```python
from build123d import *

# Parameters (mm, degrees)
SZKIC1_R                    = 85
SZKIC1_R_2                  = 70
DODANIE_WYCI_GNI_CIE1_DEPTH = 10
WYTNIJ_WYCI_GNI_CIE1_START  = -10
SZKIC2_R                    = 3.4
WYTNIJ_WYCI_GNI_CIE1_DEPTH  = 10
SZYK_KO_OWY1_COUNT          = 4


with BuildPart() as part:
    # Szkic1 → Dodanie-wyciągnięcie1 (new body)
    with BuildSketch(Plane.XY):
        Circle(SZKIC1_R)
        Circle(SZKIC1_R_2, mode=Mode.SUBTRACT)
    extrude(amount=DODANIE_WYCI_GNI_CIE1_DEPTH)

    # Szkic2 → Wytnij-wyciągnięcie1 (cut)
    with BuildSketch(Plane.XY.offset(10).offset(WYTNIJ_WYCI_GNI_CIE1_START)):
        with Locations((0, 77.5)):
            Circle(SZKIC2_R)
        with BuildLine():
            Line((-56.196738148, 53.368311023), (-61.501649853, 58.673222728))
            ThreePointArc((-61.501649853, 58.673222728), (-60.104076401, 60.104076401), (-58.673222728, 61.501649853))
            Line((-58.673222728, 61.501649853), (-53.368311023, 56.196738148))
            ThreePointArc((-53.368311023, 56.196738148), (-54.800775542, 54.800775542), (-56.196738148, 53.368311023))
        make_face()
    wytnij_wyci_gni_cie1 = extrude(amount=WYTNIJ_WYCI_GNI_CIE1_DEPTH, mode=Mode.SUBTRACT)

    # Szyk kołowy1: Wytnij-wyciągnięcie1 ×4 about axis
    szyk_ko_owy1_axis = Axis((0, 0, 0), (0, 0, 1))
    for i in range(1, SZYK_KO_OWY1_COUNT):
        add(wytnij_wyci_gni_cie1.rotate(szyk_ko_owy1_axis, i * 360 / SZYK_KO_OWY1_COUNT), mode=Mode.SUBTRACT)


solid = part.part
```
Geometry: final body of the model. Coordinates: model frame, mm. A direction names the side the tool comes from. Coordinates: 2 decimals unless noted, no trailing zeros. Order: outer loops, then holes, each group sorted by start corner. A loop starts at its lowest first (then second) coordinate and runs counter-clockwise, first axis right, second up.
Item 1: Contact query for flat-ended pins moving along their axis: P1, Ø6, axis at x = -60, z = 8.5, coming from the +Y side; P2, Ø2, axis at y = 39.5, z = 1, coming from the -X side; P3, Ø1, axis at x = 48, z = 3.5, coming from the -Y side; P4, Ø8, axis at x = -63, y = 6.5, coming from the -Z side. Output: stop coordinate, or through.
Answer:
P1: stops at y = 63.06
P2: stops at x = -75.78
P3: stops at y = -70.49
P4: passes through
Item 2: Section query D-D (x = -37). Output: boundary loops of the cut face in (y, z), then the cut area to 3 significant figures.
Answer:
outline: (-76.52, 0) - (-59.42, 0) - (-59.42, 10) - (-76.52, 10) - close; (59.42, 0) - (76.52, 0) - (76.52, 10) - (59.42, 10) - close
area: 342 mm2
Item 3: Access query for faces 4 (the face through (-56.06, 58.89, 4.93)), 5 (the face through (84.995, -0.907, 4.93)). Directions: +Z, -Z, +X, -X, +Y, -Y. A direction counts if a zero-diameter tool reaches every point of the face in a straight line with its end or side. Return the directions, or none.
Answer:
face 4: +Z, -Z
face 5: +Z, -Z, +X
Item 4: Material intervals for line 1 along Y through (x, z) = (0, 5); line 2 along Y through (x, z) = (3, 7.5); line 3 along X through (y, z) = (-61, 7.5), sorted ascending.
Answer:
line 1: y = -85 to -80.9, -74.1 to -70, 70 to 74.1, 80.9 to 85
line 2: y = -84.95 to -79.1, -75.9 to -69.94, 69.94 to 75.9, 79.1 to 84.95
line 3: x = -58.17 to -34.34, 34.34 to 58.17
Item 5: Draft query along X for faces 1 (the face through (-0.907, -84.995, 4.93)), 2 (the face through (-0.74, 74.18, 4.93)), 3 (the face through (-84.995, 0.907, 4.93)). Return one class per face: released by +X, released by -X, zero draft, split by the parting line, or undercut.
Answer:
face 1: split by the parting line
face 2: undercut
face 3: released by -X
Item 6: Section query C-C (z = 6). Output: boundary loops of the cut face in (x, y), then the cut area to 3 significant figures.
Answer:
outline: (-61.5, -58.67) - (-56.2, -53.37) arc R77.5 ccw to (-53.37, -56.2) - (-58.67, -61.5) arc R85 ccw to (58.67, -61.5) - (53.37, -56.2) arc R77.5 ccw to (56.2, -53.37) - (61.5, -58.67) arc R85 ccw to (61.5, 58.67) - (56.2, 53.37) arc R77.5 ccw to (53.37, 56.2) - (58.67, 61.5) arc R85 ccw to (-58.67, 61.5) - (-53.37, 56.2) arc R77.5 ccw to (-56.2, 53.37) - (-61.5, 58.67) arc R85 ccw to start; hole circle Ø6.8 at (-77.5, 0); hole circle Ø140 at (0, 0); hole circle Ø6.8 at (0, -77.5); hole circle Ø6.8 at (0, 77.5); hole circle Ø6.8 at (77.5, 0)
area: 7,040 mm2
Item 7: Section query A-A (x = 0). Output: boundary loops of the cut face in (y, z), then the cut area to 3 significant figures.
Answer:
outline: (-85, 0) - (-80.9, 0) - (-80.9, 10) - (-85, 10) - close; (-74.1, 0) - (-70, 0) - (-70, 10) - (-74.1, 10) - close; (70, 0) - (74.1, 0) - (74.1, 10) - (70, 10) - close; (80.9, 0) - (85, 0) - (85, 10) - (80.9, 10) - close
area: 164 mm2
